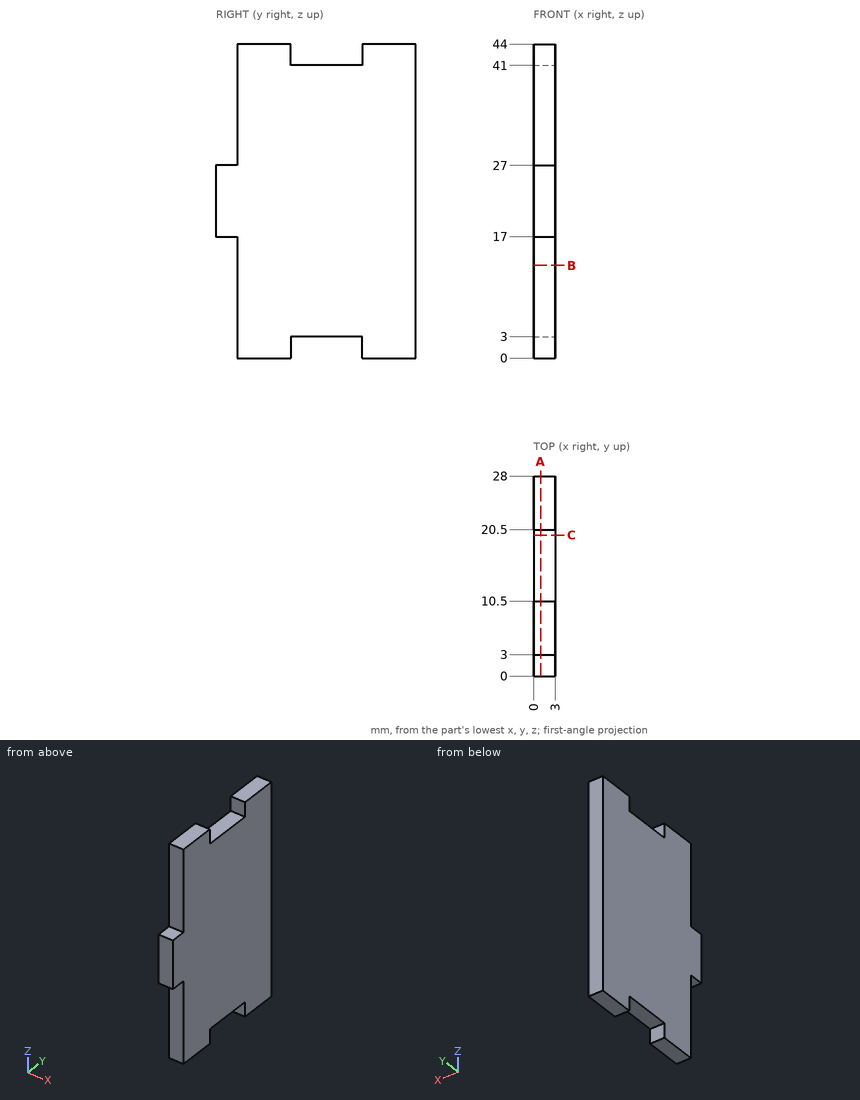
The drawing under review shows one solid part. Ordinate dimensions are in mm from its lowest x, y, z. Give positions to 0.01 mm unless a question says otherwise; leave off trailing zeros. Order: outer loops, then holes, each group sorted by start corner. A loop starts at its lowest first (then second) coordinate and runs counter-clockwise, first axis right, second up. Notation, with made-up numbers: (-28.75, 30) - (-0.75, 30) arc R23 cw to (-0.75, 68) - close; hole circle Ø1 at (-1.5, -26). An arc over 180 degrees is marked (long way). Answer as a JSON object with one key per item and string values. Group by question number.
Item 1: Clearance check with flat-ended pins moving along their axes: pin 1 Ø0.9 at (x, z) = (1.5, 43) entering from -Y; pin 2 Ø1.5 at (x, y) = (1.5, 16) entering from -Z; pin 3 Ø1.5 at (x, y) = (1.5, 2) entering from -Z. State where each tip first meets the part, or that it passes through.
Item 2: Take a section at A-A on x = 0.95. Give the boundary of the cut face in (y, z), and give its area (3 significant figures).
Item 3: Take a section at C-C on y = 19.75. Give the boundary of the cut face in (x, z).
Item 4: Wall thickness on line 1 along Z through (x, y) = (1.6, 19); line 2 along Z through (x, y) = (2.65, 2.5); line 3 along Y through (x, z) = (2.1, 5): over which ranges is each line inside the solid? List them lowest first.
Item 5: Take a section at B-B on z = 13. Give the boundary of the cut face in (x, y), and give its area (3 significant figures).
Reported:
{
 "1": {"pin 1": "y = 3", "pin 2": "z = 3", "pin 3": "z = 17"},
 "2": {"outline": "(0, 17) - (3, 17) - (3, 0) - (10.5, 0) - (10.5, 3) - (20.5, 3) - (20.5, 0) - (28, 0) - (28, 44) - (20.5, 44) - (20.5, 41) - (10.5, 41) - (10.5, 44) - (3, 44) - (3, 27) - (0, 27) - close", "area": "1,070 mm^2"},
 "3": {"outline": "(0, 3) - (3, 3) - (3, 41) - (0, 41) - close"},
 "4": {"line 1": "3 to 41", "line 2": "17 to 27", "line 3": "3 to 28"},
 "5": {"outline": "(0, 3) - (3, 3) - (3, 28) - (0, 28) - close", "area": "75.0 mm^2"}
}
